The model under review builds one solid part; all positions refer to its coordinate system, in mm. Give positions to 0.01 mm unless a question says otherwise; leave off trailing zeros. Return JSON: item names as keys, results as strings. Group by question number.
from build123d import *

# Parameters (mm, degrees)
CROQUIS1_W              = 72.5
CROQUIS1_H              = 80
CROQUIS1_R              = 1.5
CROQUIS1_R_2            = 2.5
SALIENTE_EXTRUIR1_DEPTH = 6
CHAFL_N1_SIZE           = 0.5


with BuildPart() as part:
    # Croquis1 → Saliente-Extruir1 (new body)
    with BuildSketch(Plane(origin=(0, 0, 0), x_dir=(1, 0, 0), z_dir=(0, 1, 0))):
        with Locations((5.730956658, -13.721461187)):
            Rectangle(CROQUIS1_W, CROQUIS1_H)
        with Locations(Location((16.980956658, 6.278538813, 0), (0, 0, 270))):
            Circle(CROQUIS1_R, mode=Mode.SUBTRACT)
        with Locations(Location((36.980956658, 6.278538813, 0), (0, 0, 270))):
            Circle(CROQUIS1_R, mode=Mode.SUBTRACT)
        with Locations(Location((16.980956658, -13.721461187, 0), (0, 0, 270))):
            Circle(CROQUIS1_R, mode=Mode.SUBTRACT)
        with Locations(Location((36.980956658, -13.721461187, 0), (0, 0, 270))):
            Circle(CROQUIS1_R, mode=Mode.SUBTRACT)
        with Locations(Location((-7.019043342, -3.721461187, 0), (0, 0, 270))):
            Circle(CROQUIS1_R, mode=Mode.SUBTRACT)
        with Locations(Location((4.980956658, -3.721461187, 0), (0, 0, 270))):
            Circle(CROQUIS1_R, mode=Mode.SUBTRACT)
        with Locations(Location((-22.519043342, 18.778538813, 0), (0, 0, 270))):
            Circle(CROQUIS1_R_2, mode=Mode.SUBTRACT)
        with Locations(Location((-22.519043342, -46.221461187, 0), (0, 0, 270))):
            Circle(CROQUIS1_R_2, mode=Mode.SUBTRACT)
        with Locations(Location((-19.019043342, -3.721461187, 0), (0, 0, 270))):
            Circle(CROQUIS1_R, mode=Mode.SUBTRACT)
    extrude(amount=SALIENTE_EXTRUIR1_DEPTH)

    # Chaflán1
    chafl_n1_edges = [part.edges().sort_by_distance(p)[0] for p in [
        (41.980956658, 6, 13.721461187),
        (16.980956658, 0, -7.778538813),
        (16.980956658, 6, -7.778538813),
        (5.730956658, 6, -26.278538813),
        (36.980956658, 0, -7.778538813),
        (36.980956658, 6, -7.778538813),
        (16.980956658, 0, 12.221461187),
        (16.980956658, 6, 12.221461187),
        (36.980956658, 0, 12.221461187),
        (36.980956658, 6, 12.221461187),
        (-7.019043342, 0, 2.221461187),
        (-7.019043342, 6, 2.221461187),
        (4.980956658, 0, 2.221461187),
        (4.980956658, 6, 2.221461187),
        (-22.519043342, 0, -21.278538813),
        (-22.519043342, 6, -21.278538813),
        (-22.519043342, 0, 43.721461187),
        (-22.519043342, 6, 43.721461187),
        (-30.519043342, 6, 13.721461187),
        (-19.019043342, 0, 2.221461187),
        (-19.019043342, 6, 2.221461187),
        (5.730956658, 0, -26.278538813),
        (41.980956658, 0, 13.721461187),
        (5.730956658, 0, 53.721461187),
        (-30.519043342, 0, 13.721461187),
        (5.730956658, 6, 53.721461187),
        (-30.519043342, 3, -26.278538813),
        (41.980956658, 3, -26.278538813),
        (41.980956658, 3, 53.721461187),
        (-30.519043342, 3, 53.721461187),
    ]]
    chamfer(chafl_n1_edges, length=CHAFL_N1_SIZE)


solid = part.part
Item 1: For L1, parallel to X at y = 1.25, z = 14.5; L2, parallel to X at y = 0.5, z = -18.5; L3, parallel to X at y = 1.5, z = 5, list the stretches that pass through material, from the lowest coordinate up. Write a range as from..to.
Item 2: For P1, Ø2.5, axis at x = 16.98, z = -6.28, coming from the +Y side (3 decimals); P2, Ø5, axis at x = 4.98, z = 3.72, coming from the +Y side; P3, Ø3.5, axis at x = -7.02, z = 3.72, coming from the +Y side, all flat-tipped, find the tip position at first contact; note any pin that passes through.
Item 3: Mouldability with a two-part tool opening along Z and no side actions: class faces 1 (the face through (5, 6, 13)), 2 (the face through (-20.483, 2.965, 3.396)), 3 (the face through (5, 3, 53.721)) as +Z half, -Z half, draft (parallel to the pull), parting line (faces both ways), or undercut.
Item 4: Take a section at A-A (y = 3.25). State how many separate pieces and enclosed holes the cut face has, then the cut area to 3 significant figures.
Check sheet entries:
{
 "1": {"L1": "x = -30.52..15.7, 18.26..35.7, 38.26..41.98", "L2": "x = -30.52..-25, -20.03..41.98", "L3": "x = -30.52..-19.8, -18.23..-7.8, -6.23..4.2, 5.77..41.98"},
 "2": {"P1": "passes through", "P2": "stops at y = 6", "P3": "stops at y = 5.75"},
 "3": {"face 1": "draft", "face 2": "undercut", "face 3": "+Z half"},
 "4": {"separate pieces": "1", "enclosed holes": "9", "area": "5,710 mm^2"}
}
